The listing builds one solid part. Answer for the finished solid, in the listing's coordinates (mm). Give positions to 0.01 mm unless a question says otherwise; leave off trailing zeros. Write each loop counter-clockwise with the first axis right and the second up, starting at its lowest first coordinate (ties: lowest second). Pieces come first, ordered by that corner, then holes. Notation, with made-up numbers: (-26, 87) - (-21, 87) arc R34 ccw to (-21, 121) - close; hole circle Ø6 at (56, -1). An arc over 180 degrees is marked (long way). Answer as CSV lines item,"result". Start each with the question number.
(1) Each of these flat-tipped pins is pushed along its axis until it touches: pin 1 Ø12 at (x, y) = (983, 258.5) entering from +Z; pin 2 Ø2 at (x, y) = (975, 313.5) entering from -Z; pin 3 Ø6 at (x, y) = (958.5, -306) entering from -Z. Where does it stop, or does it pass through?
(2) Straight lines are drawn through the part: probe 1 along Y at (x, z) = (953, 467.5); probe 2 along Y at (x, z) = (978.5, 693.5); probe 3 along Z at (x, y) = (984, 134.5). For each, find the intervals that lie inside material, in ascending order.
(3) Find section C-C (x = 987). Write down the section's boundary in (y, z).
(4) Find section B-B (y = 324.5). Write down the section's boundary in (x, z), then the cut area to 3 significant figures.
(5) Find section A-A (z = 855). Write down the section's boundary in (x, y).
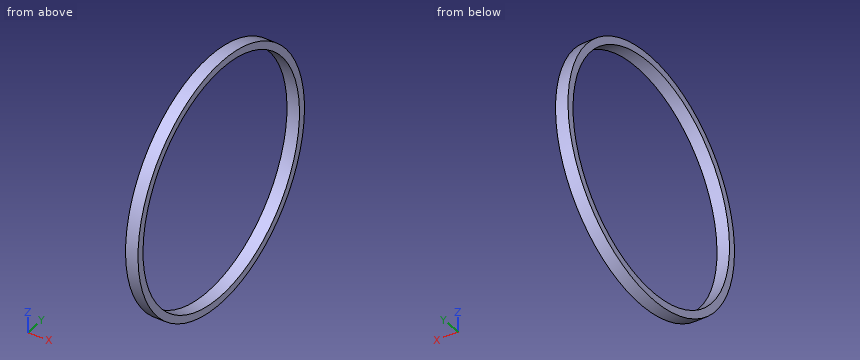
from build123d import *

# Parameters (mm, degrees)
CYLINDER001_R     = 470
CYLINDER001_DEPTH = 50
CYLINDER002_R     = 500
CYLINDER002_DEPTH = 50


with BuildPart() as cilindro001:
    # Cylinder001 → Cylinder001 (new body)
    with BuildSketch(Plane(origin=(1000, 0, 465.754524), x_dir=(0, 0, 1), z_dir=(-1, 0, 0))):
        Circle(CYLINDER001_R)
    extrude(amount=CYLINDER001_DEPTH)


with BuildPart() as cut:
    # Cylinder002 → Cylinder002 (new body)
    with BuildSketch(Plane(origin=(1000, 0, 465.754524), x_dir=(0, 0, 1), z_dir=(-1, 0, 0))):
        Circle(CYLINDER002_R)
    extrude(amount=CYLINDER002_DEPTH)

    # Cut: cut Cilindro001
    add(cilindro001.part, mode=Mode.SUBTRACT)


solid = cut.part
Result set:
1,pin 1,"z = 897.31"
1,pin 2,"z = 75.44"
1,pin 3,"z = 68.02"
2,probe 1,"-500 to -470, 470 to 500"
2,probe 2,"-445.12 to -411.14, 411.14 to 445.12"
2,probe 3,"-15.82 to 15.41, 916.1 to 947.32"
3,outline,"circle Ø1000 at (0, 465.75); hole circle Ø940 at (0, 465.75)"
4,outline,"(950, 85.36) - (1000, 85.36) - (1000, 125.75) - (950, 125.75) - close; (950, 805.75) - (1000, 805.75) - (1000, 846.15) - (950, 846.15) - close"
4,area,"4,040 mm^2"
5,outline,"(950, -313.83) - (1000, -313.83) - (1000, -263.42) - (950, -263.42) - close; (950, 263.42) - (1000, 263.42) - (1000, 313.83) - (950, 313.83) - close"
